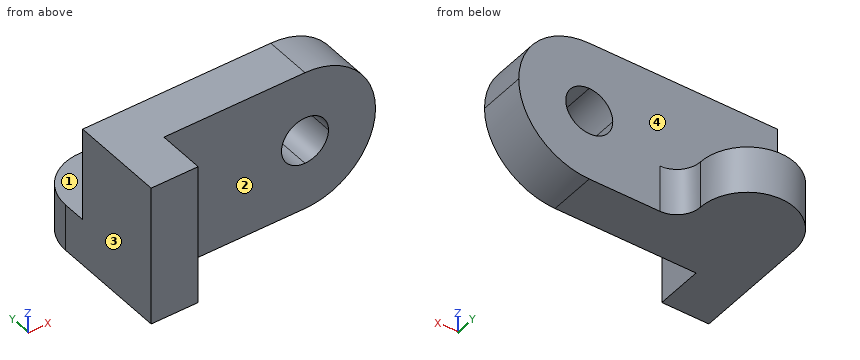
from build123d import *

# Parameters (mm, degrees)
F1_DEPTH = 12.7
F2_W     = 12.7
F2_H     = 19.05
F3_DEPTH = 12.7
F4_W     = 31.75
F4_H     = 12.7
F5_DEPTH = 6.35
F6_R     = 6.35
F7_DEPTH = 25.4
F9_DEPTH = 12.7


with BuildPart() as f1:
    # F0 (on Front) → F1 (new body)
    with BuildSketch(Plane.XZ):
        with BuildLine():
            ThreePointArc((0, -19.05), (-13.4703841816, -13.4703841816), (-19.05, 0))
            Line((-19.05, 0), (-50.8, 0))
            Line((-50.8, 0), (-50.8, -19.05))
            Line((-50.8, -19.05), (0, -19.05))
        make_face()
        with BuildLine():
            ThreePointArc((0, 19.05), (-13.4703841816, 13.4703841816), (-19.05, 0))
            Line((-19.05, 0), (-6.35, 0))
            ThreePointArc((-6.35, 0), (-4.4901280605, 4.4901280605), (0, 6.35))
            Line((0, 6.35), (0, 19.05))
        make_face()
        with BuildLine():
            Line((-50.8, 0), (-19.05, 0))
            ThreePointArc((-19.05, 0), (-13.4703841816, 13.4703841816), (0, 19.05))
            Line((0, 19.05), (-50.8, 19.05))
            Line((-50.8, 19.05), (-50.8, 0))
        make_face()
        with BuildLine():
            Line((-6.35, 0), (-19.05, 0))
            ThreePointArc((-19.05, 0), (-13.4703841816, -13.4703841816), (0, -19.05))
            Line((0, -19.05), (0, -6.35))
            ThreePointArc((0, -6.35), (-4.4901280605, -4.4901280605), (-6.35, 0))
        make_face()
        with BuildLine():
            ThreePointArc((19.05, 0), (13.4703841816, 13.4703841816), (0, 19.05))
            Line((0, 19.05), (0, 6.35))
            ThreePointArc((0, 6.35), (4.4901280605, 4.4901280605), (6.35, 0))
            Line((6.35, 0), (19.05, 0))
        make_face()
        with BuildLine():
            Line((0, -6.35), (0, -19.05))
            ThreePointArc((0, -19.05), (13.4703841816, -13.4703841816), (19.05, 0))
            Line((19.05, 0), (6.35, 0))
            ThreePointArc((6.35, 0), (4.4901280605, -4.4901280605), (0, -6.35))
        make_face()
    extrude(amount=F1_DEPTH)

    # F2 (on face) → F3 (join)
    with BuildSketch(Plane.XZ.offset(12.7)):
        with Locations((-44.45, -9.525)):
            Rectangle(F2_W, F2_H)
        with Locations((-44.45, 9.525)):
            Rectangle(F2_W, F2_H)
    extrude(amount=F3_DEPTH)

    # F4 (on face) → F5 (join)
    with BuildSketch(Plane(origin=(0, 0, 0), x_dir=(-1, 0, 0), z_dir=(0, 1, 0))):
        with Locations((34.925, -12.7)):
            Rectangle(F4_W, F4_H)
    extrude(amount=F5_DEPTH)

    # F6 (on face) → F7 (cut)
    with BuildSketch(Plane.XY.offset(-6.35)):
        with Locations((-19.05, 6.35)):
            Circle(F6_R)
    extrude(amount=-F7_DEPTH, mode=Mode.SUBTRACT)

    # F8 (on face) → F9 (join)
    with BuildSketch(Plane.XY.offset(-6.35)):
        with BuildLine():
            ThreePointArc((-25.4, 6.35), (-38.1, 19.05), (-50.8, 6.35))
            Line((-50.8, 6.35), (-38.1, 6.35))
            Line((-38.1, 6.35), (-25.4, 6.35))
        make_face()
    extrude(amount=-F9_DEPTH)


solid = f1.part
Verification items for the finished model (mm, model axes). Face numbers are marked on the shaded views. A direction names the side the tool comes from. Give positions to 0.01 mm unless a question says otherwise; leave off trailing zeros. Order: outer loops, then holes, each group sorted by start corner. A loop starts at its lowest first (then second) coordinate and runs counter-clockwise, first axis right, second up. Notation, with made-up numbers: M 71,54.5 L 94,54.5 A24 ccw 94,64.5 Z; hole C 25,42 d10. An arc over 180 degrees is marked long. Answer as a JSON object with one key per item and string values. Group by question number.
1) Cross-section at D-D (y = -18.5). Enter the section's corners in (x, z), then the cut area to 3 significant figures.
2) Cross-section at C-C (x = -43). Enter the section's corners in (y, z), then the cut area to 3 significant figures.
3) Cross-section at B-B (z = -2.5). Enter the section's corners in (x, y), then the cut area to 3 significant figures.
4) Cross-section at A-A (y = -10). Enter the section's corners in (x, z), then the cut area to 3 significant figures.
5) Scan lines: line 1 along Y through (x, z) = (-7.5, 4); line 2 along X through (y, z) = (-15, -5); line 3 along X through (y, z) = (-8, 5). Record each from-to range of solid material in increasing order. Write a range as [from, to].
6) Depth check by flat-ended pin: pin 1 Ø4 at (x, z) = (-28.5, -2) entering from -Y; pin 2 Ø9.5 at (x, y) = (-32, 8) entering from +Z; pin 3 Ø1.5 at (x, z) = (9.5, -12) entering from +Y. Enter the tip coordinate at first touch or a pass-through.
7) Access from +Z, -Z, +X, -X, +Y, -Y to the whole of each face (thin tool, end or side, straight path). Record for the marked faces 1, 2, 3 and 4.
Result sheet:
{
 "1": {"outline": "M -50.8,-19.05 L -38.1,-19.05 L -38.1,19.05 L -50.8,19.05 Z", "area": "484 mm2"},
 "2": {"outline": "M -25.4,-19.05 L 18.07,-19.05 L 18.07,-6.35 L 0,-6.35 L 0,19.05 L -25.4,19.05 Z", "area": "1,200 mm2"},
 "3": {"outline": "M -50.8,-25.4 L -38.1,-25.4 L -38.1,-12.7 L -5.84,-12.7 L -5.84,0 L -50.8,0 Z; M 5.84,-12.7 L 18.89,-12.7 L 18.89,0 L 5.84,0 Z", "area": "898 mm2"},
 "4": {"outline": "M -50.8,-19.05 L 0,-19.05 A19.05 ccw 0,19.05 L -50.8,19.05 Z; hole C 0,0 d12.7", "area": "2,380 mm2"},
 "5": {"line 1": "y = [-12.7, 0]", "line 2": "x = [-50.8, -38.1]", "line 3": "x = [-50.8, -3.91], [3.91, 18.38]"},
 "6": {"pin 1": "stops at y = -12.7", "pin 2": "stops at z = -6.35", "pin 3": "stops at y = 0"},
 "7": {"face 1": "+Z, +X, -X, +Y", "face 2": "+Z, -Z, +X, -Y", "face 3": "+Z, -Z, -X, +Y, -Y", "face 4": "+Z, +X, +Y"}
}
